Design review of the part built by this model. Coordinates are the model's own, in mm. Coordinates: 2 decimals unless noted, no trailing zeros. Order: outer loops, then holes, each group sorted by start corner. A loop starts at its lowest first (then second) coordinate and runs counter-clockwise, first axis right, second up. Notation, with made-up numbers: M 65,-16 L 92,-16 A35 ccw 92,20 Z; hole C -21.5,-7 d6. An arc over 180 degrees is marked long. Use CSV: the item, a comma, the result in double quotes.
```python
from build123d import *

# Parameters (mm, degrees)
ENL_V_MAT_EXTRU_1_DEPTH      = 7.5
ENL_V_MAT_EXTRU_1_DEPTH_BACK = 7.5
BOSS_EXTRU_1_REACH           = 27.5
ECHELLE1_SCALE               = 2


with BuildPart() as part:
    # Esquisse1 → R_volution1 (revolve)
    with BuildSketch(Plane.XY):
        with BuildLine():
            Line((0, 0), (0, 100))
            Line((0, 100), (-18, 100))
            Line((-18, 100), (-7.593007693, 6.792401612))
            ThreePointArc((-7.593007693, 6.792401612), (-5.093880777, 1.945904787), (0, 0))
        make_face()
    revolve(axis=Axis((0, 0, 0), (0, 1, 0)))

    # Esquisse2 → Enl_v. mat.-Extru.1 (cut, two sides)
    with BuildSketch(Plane.XY) as enl_v_mat_extru_1_sk:
        with BuildLine():
            Line((-13.5, 100), (13.5, 100))
            add(Edge.make_bspline(
                [(-13.5, 100), (-13.291113541, 83.520875666), (13.291113541, 83.520875666), (13.5, 100)],
                knots=[0, 0, 0, 0, 1, 1, 1, 1], degree=3))
        make_face()
    extrude(amount=ENL_V_MAT_EXTRU_1_DEPTH, mode=Mode.SUBTRACT)
    extrude(enl_v_mat_extru_1_sk.sketch, amount=-ENL_V_MAT_EXTRU_1_DEPTH_BACK, mode=Mode.SUBTRACT)

    # Esquisse3 → Boss.-Extru.1 (add, up to next)
    with BuildSketch(Plane.XY.offset(-7.5), mode=Mode.PRIVATE) as boss_extru_1_sk1:
        with BuildLine():
            Line((-5, 100), (5, 100))
            add(Edge.make_bspline(
                [(-5, 100), (0, 91.498247822), (5, 100)],
                knots=[0, 0, 0, 1, 1, 1], degree=2))
        make_face()
    boss_extru_1_tool1 = extrude(boss_extru_1_sk1.sketch, amount=BOSS_EXTRU_1_REACH, mode=Mode.PRIVATE) - part.part
    add(boss_extru_1_tool1.solids().sort_by_distance((0, 98.29965, -7.5))[0])


with BuildPart() as part_1:
    # Echelle1: scaled about (-4e-09, 62.219241992, 3e-09)
    add(part.part.scale(ECHELLE1_SCALE).moved(Location((4e-09, -62.219241992, -3e-09))))


solid = part_1.part
```
(1) Wall thickness on probe 1 along X at (y, z) = (-45, -3.5); probe 2 along X at (y, z) = (38.5, 16); probe 3 along Z at (x, y) = (-26.5, 116): over which ranges is each line inside the solid? List them lowest first.
The answers:
probe 1,"x = -15.19 to 15.19"
probe 2,"x = -19.1 to 19.1"
probe 3,"z = -20.61 to 20.61"
(2) Add section A-A on y = -46. State the section outline as (x, z) points.
The answers:
outline,"C 0,0 d30.96"
(3) Add section B-B on y = 26. State the section outline as (x, z) points.
The answers:
outline,"C 0,0 d47.04"
(4) The part is to be moulded in two halves that separate along Y. For faces 1 (the face through (-1, 137.781, 1)), 2 (the face through (0, 125, -15)), 3 (the face through (20.194, 43.268, -15.484)), say which applies: pulls with the +Y half, pulls with the -Y half, needs draft (parallel to the pull), parting line crosses it, or undercut.
The answers:
face 1,"pulls with the +Y half"
face 2,"undercut"
face 3,"pulls with the -Y half"
(5) Clearance check with flat-ended pins moving along their axes: P1, Ø2, axis at y = 4, z = 7, coming from the -X side; P2, Ø1.5, axis at y = 77.5, z = -5, coming from the -X side; P3, Ø5, axis at y = 19, z = 1.5, coming from the -X side. State where each tip first meets the part, or that it passes through.
The answers:
P1,"stops at x = -20.21"
P2,"stops at x = -28.99"
P3,"stops at x = -22.99"
